Model file for the job. Use its own axes, mm. A direction names the side the tool comes from. Round coordinates to 2 decimals unless told otherwise and drop trailing zeros. Loops run counter-clockwise (first coordinate to the right, second up) from the corner with the lowest first, then second, coordinate; pieces in that order, holes last. Notation, with made-up numbers: (-34, -6.75) -> (-8, -6.75) arc R29 cw to (-8, 22.25) -> close; hole circle Ø4 at (-3, 24). An arc over 180 degrees is marked (long way). Use a Markdown table: item, result. Add a question column.
```python
from build123d import *

# Parameters (mm, degrees)
SKETCH_1_W      = 34
SKETCH_1_H      = 14
SKETCH_1_R      = 5.05
SKETCH_1_W_2    = 5
SKETCH_1_H_2    = 5
EXTRUDE_1_DEPTH = 10


with BuildPart() as part:
    # 草图1 → 凸台-拉伸1 (new body)
    with BuildSketch(Plane.XY):
        Rectangle(SKETCH_1_W, SKETCH_1_H)
        with Locations((-10, 0)):
            Circle(SKETCH_1_R, mode=Mode.SUBTRACT)
        with Locations((10, 0)):
            Circle(SKETCH_1_R, mode=Mode.SUBTRACT)
        Rectangle(SKETCH_1_W_2, SKETCH_1_H_2, mode=Mode.SUBTRACT)
    extrude(amount=EXTRUDE_1_DEPTH)


solid = part.part
```
1) Cut at C-C on z = 4.25. Write the cut outline in (x, y), and give its area (3 significant figures).
2) Tool access for faces 5 (the face through (-2.5, 0, 5)), 6 (the face through (0, 3, 0)): list every direction of +Z, -Z, +X, -X, +Y, -Y with a clear straight run to the whole face (end or side of a thin tool).
3) Cut at A-A on y = 0. Write the cut outline in (x, z).
4) Cut at D-D on x = -8.5. Write the cut outline in (y, z), and give its area (3 significant figures).
5) Pull direction Y, two halves, no side cores. Call faces 1 (the face through (0, 7, 5)), 2 (the face through (0, -2.5, 5)), 3 (the face through (2.5, 0, 5)), 4 (the face through (0, -7, 5)): +Y half, -Y half, draft (parallel to the pull), parting line (faces both ways), or undercut.
6) Wall check: probe 1 along Y at (x, z) = (10, 5); probe 2 along X at (y, z) = (1.75, 9.25); probe 3 along Y at (x, z) = (-11, 2.25). Give the ranges that are in metal, low to high. Write a range as from..to.
7) Cut at B-B on x = 10. Write the cut outline in (y, z), and give its area (3 significant figures).
Established:
| question | item | result |
|---|---|---|
| 1 | outline | (-17, -7) -> (17, -7) -> (17, 7) -> (-17, 7) -> close; hole circle Ø10.1 at (-10, 0); hole (-2.5, -2.5) -> (2.5, -2.5) -> (2.5, 2.5) -> (-2.5, 2.5) -> close; hole circle Ø10.1 at (10, 0) |
| 1 | area | 291 mm^2 |
| 2 | face 5 | +Z, -Z |
| 2 | face 6 | -Z, +X, -X, +Y, -Y |
| 3 | outline | (-17, 0) -> (-15.05, 0) -> (-15.05, 10) -> (-17, 10) -> close; (-4.95, 0) -> (-2.5, 0) -> (-2.5, 10) -> (-4.95, 10) -> close; (2.5, 0) -> (4.95, 0) -> (4.95, 10) -> (2.5, 10) -> close; (15.05, 0) -> (17, 0) -> (17, 10) -> (15.05, 10) -> close |
| 4 | outline | (-7, 0) -> (-4.82, 0) -> (-4.82, 10) -> (-7, 10) -> close; (4.82, 0) -> (7, 0) -> (7, 10) -> (4.82, 10) -> close |
| 4 | area | 43.6 mm^2 |
| 5 | face 1 | +Y half |
| 5 | face 2 | undercut |
| 5 | face 3 | undercut |
| 5 | face 4 | -Y half |
| 6 | probe 1 | y = -7..-5.05, 5.05..7 |
| 6 | probe 2 | x = -17..-14.74, -5.26..-2.5, 2.5..5.26, 14.74..17 |
| 6 | probe 3 | y = -7..-4.95, 4.95..7 |
| 7 | outline | (-7, 0) -> (-5.05, 0) -> (-5.05, 10) -> (-7, 10) -> close; (5.05, 0) -> (7, 0) -> (7, 10) -> (5.05, 10) -> close |
| 7 | area | 39.0 mm^2 |
